from build123d import *

# Parameters (mm, degrees)
REVOLVE1_ANGLE = 180
SKETCH2_R      = 3
EXTRUDE1_DEPTH = 40
EXTRUDE1_TAPER = 1


with BuildPart() as part:
    # Sketch1 → Revolve1 (revolve)
    with BuildSketch(Plane.XY):
        with BuildLine():
            Line((-20, 0), (20, 0))
            ThreePointArc((20, 0), (19.267766953, 1.767766953), (17.5, 2.5))
            Line((17.5, 2.5), (-17.5, 2.5))
            ThreePointArc((-17.5, 2.5), (-19.267766953, 1.767766953), (-20, 0))
        make_face()
    revolve(axis=Axis((-20, 0, 0), (1, 0, 0)), revolution_arc=REVOLVE1_ANGLE)

    # Sketch2 → Extrude1 (add)
    with BuildSketch(Plane(origin=(0, 0, 0), x_dir=(-1, 0, 0), z_dir=(0, 0, -1))):
        Circle(SKETCH2_R)
    extrude(amount=-EXTRUDE1_DEPTH, taper=EXTRUDE1_TAPER)


solid = part.part
For this review, take the finished solid that the model builds, in its own axes (mm). A direction names the side the tool comes from. Round coordinates to 2 decimals unless told otherwise and drop trailing zeros. Loops run counter-clockwise (first coordinate to the right, second up) from the corner with the lowest first, then second, coordinate; pieces in that order, holes last. Notation, with made-up numbers: (-27.75, 71) - (7.25, 71) arc R16 ccw to (7.25, 94) - close; hole circle Ø8 at (1.25, 76.5). An arc over 180 degrees is marked (long way). Put each result on its own line as item: value. Start each with the question number.
1. For probe 1 along Z at (x, y) = (12, -1); probe 2 along Z at (x, y) = (-6.5, -1.25); probe 3 along X at (y, z) = (-0.25, 26), list the stretches that pass through material, from the lowest coordinate up. Write a range as [from, to].
2. For faces 1 (the cylindrical face through (-9.7, 0.1, 2.5)), 2 (the cylindrical face through (9.5, 0.1, 2.5)), 3 (the conical face through (2.1, -1.61, 20.28)), 4 (the flat face through (0, 0, 40)), list the 3-axis set-ups (+Z, -Z, +X, -X, +Y, -Y) from which the entire face can be reached by the end or side of a thin tool; tool diameter is ignored.
3. Consider section D-D on x = -13. State the section outline as (y, z) points, plus the area to 3 significant figures.
4. Insertion check: P1, Ø3, axis at y = -1, z = 33.5, coming from the -X side; P2, Ø3, axis at y = 1.5, z = 6.5, coming from the +X side; P3, Ø3, axis at y = 0, z = 28.5, coming from the +X side. Each pin has a flat end and moves straight along its axis. Give the tip position at first contact, or say it passes through.
5. Consider section B-B on x = 18.5. State the section outline as (y, z) points.
6. Consider section A-A on z = 12.5. State the section outline as (x, y) points, plus the area to 3 significant figures.
7. Consider section C-C on z = 27. State the section outline as (x, y) points, plus the area to 3 significant figures.
Result sheet:
1. probe 1: [0, 2.29]
1. probe 2: [0, 2.17]
1. probe 3: [-2.53, 2.53]
2. face 1: +Z, -X
2. face 2: +Z, +X
2. face 3: +Z
2. face 4: +Z, +X, -X, +Y, -Y
3. outline: (-2.5, 0) - (2.5, 0) arc R2.5 ccw to start
3. area: 9.82 mm^2
4. P1: x = -2.44
4. P2: x = 2.89
4. P3: x = 2.53
5. outline: (-2.29, 0) - (2.29, 0) arc R2.29 ccw to start
6. outline: circle Ø5.56 at (0, 0)
6. area: 24.3 mm^2
7. outline: circle Ø5.06 at (0, 0)
7. area: 20.1 mm^2
